Geometry check sheet. Reference: the model listing, model coordinates, mm. A direction names the side the tool comes from. Coordinates: 2 decimals unless noted, no trailing zeros. Order: outer loops, then holes, each group sorted by start corner. A loop starts at its lowest first (then second) coordinate and runs counter-clockwise, first axis right, second up. Notation, with made-up numbers: (29, -30.75) -> (83, -30.75) arc R9 ccw to (83, -26.75) -> close; hole circle Ø3 at (23.5, -22). An arc over 180 degrees is marked (long way). Answer in a Markdown table with one row per item. Add a question column.
```python
from build123d import *

# Parameters (mm, degrees)
SKETCH1_W           = 12.538434267
SKETCH1_H           = 35
BOSS_EXTRUDE1_DEPTH = 4
SKETCH2_W           = 2.538434267
SKETCH2_H           = 21
CUT_EXTRUDE1_DEPTH  = 37.619666847
SKETCH3_W           = 2.5
SKETCH3_H           = 21
CUT_EXTRUDE2_DEPTH  = 37.619666847
CUT_EXTRUDE3_DEPTH  = 37.619666847
SKETCH5_W           = 7.5
SKETCH5_H           = 1.65
SKETCH6_W           = 7.5
SKETCH6_H           = 1.65
HOLE1_D             = 2.013
FILLET1_R           = 1.25
SKETCH9_W           = 12.538434267
SKETCH9_H           = 7
BOSS_EXTRUDE2_DEPTH = 1


with BuildPart() as part:
    # Sketch1 → Boss-Extrude1 (new body)
    with BuildSketch(Plane(origin=(0, 0, 0), x_dir=(-1, 0, 0), z_dir=(0, 0, -1))):
        with Locations((3.730782867, 17.5)):
            Rectangle(SKETCH1_W, SKETCH1_H)
    extrude(amount=-BOSS_EXTRUDE1_DEPTH)

    # Sketch2 → Cut-Extrude1 (cut, through all)
    with BuildSketch(Plane.XY.offset(4)):
        with Locations((1.269217133, 17.5)):
            Rectangle(SKETCH2_W, SKETCH2_H)
    extrude(amount=-CUT_EXTRUDE1_DEPTH, mode=Mode.SUBTRACT)

    # Sketch3 → Cut-Extrude2 (cut, through all)
    with BuildSketch(Plane.XY.offset(4)):
        with Locations((-8.75, 17.5)):
            Rectangle(SKETCH3_W, SKETCH3_H)
    extrude(amount=-CUT_EXTRUDE2_DEPTH, mode=Mode.SUBTRACT)

    # Sketch4 → Cut-Extrude3 (cut, through all)
    with BuildSketch(Plane(origin=(0, 0, 0), x_dir=(0, 0, -1), z_dir=(1, 0, 0))):
        with BuildLine():
            Line((-2.855933763, 23.21436986), (-2.855933763, 11.78563014))
            ThreePointArc((-2.855933763, 11.78563014), (-1.992824856, 12.024984399), (-1.13183027, 11.778132681))
            Line((-1.13183027, 11.778132681), (-1.13183027, 23.221867319))
            ThreePointArc((-1.13183027, 23.221867319), (-1.992824856, 22.975015601), (-2.855933763, 23.21436986))
        make_face()
    extrude(amount=-CUT_EXTRUDE3_DEPTH, mode=Mode.SUBTRACT)

    # Sketch5 → Cut-Revolve1 (revolve, cut)
    with BuildSketch(Plane.XY.offset(2)):
        with Locations((-3.75, 11.2)):
            Rectangle(SKETCH5_W, SKETCH5_H)
    revolve(axis=Axis((-7.5, 10.375, 2), (1, 0, 0)), mode=Mode.SUBTRACT)

    # Sketch6 → Cut-Revolve2 (revolve, cut)
    with BuildSketch(Plane.XY.offset(2)):
        with Locations((-3.75, 25.45)):
            Rectangle(SKETCH6_W, SKETCH6_H)
    revolve(axis=Axis((-7.5, 24.625, 2), (1, 0, 0)), mode=Mode.SUBTRACT)

    # Hole1 (through all)
    with Locations(Plane(origin=(0, 0, 0), x_dir=(-1, 0, 0), z_dir=(0, 0, -1))):
        with Locations((0.730782866, 3.5), (6.730782866, 3.5), (0.730782866, 31.5), (6.730782866, 31.5)):
            Hole(HOLE1_D / 2)

    # Fillet1
    fillet1_edges = [part.edges().sort_by_distance(p)[0] for p in [
        (0, 7, 2),
        (0, 28, 2),
        (-7.5, 28, 2),
        (-7.5, 7, 2),
    ]]
    fillet(fillet1_edges, radius=FILLET1_R)

    # Sketch9 → Boss-Extrude2 (add)
    with BuildSketch(Plane(origin=(0, 0, 0), x_dir=(-1, 0, 0), z_dir=(0, 0, -1))):
        with Locations((3.730782867, 3.5)):
            Rectangle(SKETCH9_W, SKETCH9_H)
    extrude(amount=BOSS_EXTRUDE2_DEPTH)


solid = part.part
```
(1) Cross-section at A-A (z = 2). Give the number of separate pieces and of enclosed holes in the cut face, plus the area to 3 significant figures.
(2) Cross-section at C-C (y = 31.5). Enter the section's corners in (x, z).
(3) Access from +Z, -Z, +X, -X, +Y, -Y to the whole of each face (thin tool, end or side, straight path). Record for faces 1 (the face through (-4, 18, 2.856)), 2 (the face through (-0.19, 4.35, 2.03)), 3 (the face through (-3.6, 7, -0.7)), 4 (the face through (2, 28, 2)).
(4) Mould release check, pull along Y, two halves, no side actions. Record for faces 5 (the face through (-4, 18, 4)), 6 (the face through (0.376, 7.356, 1.972)), 7 (the face through (-4, 35, 2)): +Y half, -Y half, draft (parallel to the pull), parting line (faces both ways), or undercut.
(5) Scan lines: line 1 along Z through (x, y) = (-3.75, 19.5); line 2 along Y through (x, z) = (-3.75, 2) (3 decimals); line 3 along Y through (x, z) = (1.75, 3.2). Record each from-to range of solid material in increasing order.
(6) Go/stop test with flat-tipped pins: P1, Ø2.5, axis at y = 10.375, z = 2, coming from the +X side; P2, Ø0.6, axis at x = -0.5, y = 3, coming from the +Z side; P3, Ø2, axis at x = -4.5, y = 17.5, coming from the -Z side; P4, Ø3, axis at y = 15, z = 2.5, coming from the -X side. Record where each tip stops, or that it passes through.
(7) Cross-section at D-D (x = -4.5). Enter the section's corners in (y, z) (3 decimals), plus the area to 3 significant figures.
(8) Cross-section at B-B (y = 20). Enter the section's corners in (x, z).
Checks:
| question | item | result |
|---|---|---|
| 1 | separate pieces | 2 |
| 1 | enclosed holes | 4 |
| 1 | area | 190 mm² |
| 2 | outline | (-10, 0) -> (-7.74, 0) -> (-7.74, 4) -> (-10, 4) -> close; (-5.72, 0) -> (-1.74, 0) -> (-1.74, 4) -> (-5.72, 4) -> close; (0.28, 0) -> (2.54, 0) -> (2.54, 4) -> (0.28, 4) -> close |
| 3 | face 1 | +X, -X |
| 3 | face 2 | +Z |
| 3 | face 3 | -Z |
| 3 | face 4 | +Z, -Z, +X |
| 4 | face 5 | draft |
| 4 | face 6 | undercut |
| 4 | face 7 | +Y half |
| 5 | line 1 | 0 to 1.13, 2.86 to 4 |
| 5 | line 2 | 0 to 8.725, 26.275 to 35 |
| 5 | line 3 | 0 to 7, 28 to 35 |
| 6 | P1 | through |
| 6 | P2 | z = 0 |
| 6 | P3 | z = 0 |
| 6 | P4 | x = -7.5 |
| 7 | outline | (0, -1) -> (7, -1) -> (7, 0) -> (35, 0) -> (35, 4) -> (0, 4) -> close; hole (11.778, 1.132) -> (23.222, 1.132) arc R1.65 ccw (long way) to (23.214, 2.856) -> (11.786, 2.856) arc R1.65 ccw (long way) to start |
| 7 | area | 111 mm² |
| 8 | outline | (-7.5, 0) -> (0, 0) -> (0, 1.13) -> (-7.5, 1.13) -> close; (-7.5, 2.86) -> (0, 2.86) -> (0, 4) -> (-7.5, 4) -> close |
